For this review, take the finished solid that the model builds, in its own axes (mm). A direction names the side the tool comes from. Round coordinates to 2 decimals unless told otherwise and drop trailing zeros. Write each loop counter-clockwise with the first axis right and the second up, starting at its lowest first coordinate (ties: lowest second). Pieces come first, ordered by that corner, then holes. Notation, with made-up numbers: (21, 82) -> (55, 82) arc R19 cw to (55, 96) -> close; hole circle Ø5 at (-35.5, -8). An arc over 180 degrees is marked (long way). Answer as CSV lines item,"result". Start each with the question number.
Item 1: Take a section at B-B on y = 3.5. Give the boundary of the cut face in (x, z).
Item 2: Mouldability with a two-part tool opening along Y and no side actions: class faces 6 (the cylindrical face through (-2.38, -0.01, 7.13)), 7 (the flat face through (0, 0, 9.525)), 8 (the flat face through (3, -0.635, 8)), 9 (the cylindrical face through (-0.2, -1.51, 2.54)) as +Y half, -Y half, draft (parallel to the pull), parting line (faces both ways), or undercut.
Item 3: For pin 1 Ø0.9 at (x, z) = (3.5, 8.5) entering from -Y (3 decimals); pin 2 Ø1.5 at (x, y) = (3, -2) entering from +Z; pin 3 Ø0.9 at (x, z) = (3, 7.5) entering from +Y (3 decimals), all flat-tipped, find the tip position at first contact; note any pin that passes through.
Item 4: Machinability: for faces 1 (the flat face through (0, 0, 5.159)), 2 (the flat face through (3, 0.635, 8)), 3 (the flat face through (-3, 0.635, 8)), 4 (the flat face through (-3, -0.635, 8)), 5 (the cylindrical face through (2.38, 0.01, 7.13)), which of the approach directions +Z, -Z, +X, -X, +Y, -Y give a long, thin tool a straight path to every point of the face, cutting with its end or side? Answer none if there is none.
Item 5: Wall thickness on probe 1 along Y at (x, z) = (0, 3.55) (3 decimals); probe 2 along Z at (x, y) = (3, 2); probe 3 along Z at (x, y) = (0, 2.5): over which ranges is each line inside the solid? List them lowest first. Write a range as from..to.
```python
from build123d import *
from build123d import SkipClean  # not in build123d's __all__

# Parameters (mm, degrees)
F0_R      = 4.15
F1_DEPTH  = 1.5875
F3_R      = 4.15
F4_DEPTH  = 1.5875
F6_R      = 2.38125
F7_DEPTH  = 1.5875
F9_DEPTH  = 3.175
F10_R     = 3.175
F11_DEPTH = 3.175
F12_R     = 1.524
F13_DEPTH = 5.159375


# Not quite as in the source:
# - after a boolean that leaves OpenCascade's solid faulty, fix() repairs it


with BuildPart() as f1:
    # F0 (on Top) → F1 (new body)
    with BuildSketch(Plane.XY):
        Circle(F0_R)
    extrude(amount=F1_DEPTH)



with BuildPart() as f4:
    # F3 (on offset) → F4 (new body)
    with BuildSketch(Plane.XY.offset(6.35)):
        Circle(F3_R)
    extrude(amount=-F4_DEPTH)



with BuildPart() as f7:
    # F6 (on offset) → F7 (new body)
    with BuildSketch(Plane.XY.offset(7.9375)):
        Circle(F6_R)
    extrude(amount=F7_DEPTH)


with BuildPart() as f4_1:
    add(f4.part, clean=False)

    add(f7.part)  # F9 merges F7
    # F8 (on face) → F9 (join, through all)
    with BuildSketch(Plane.XY.offset(6.35)):
        with BuildLine():
            Line((2.2950221268, -0.635), (4.1011309416, -0.635))
            ThreePointArc((4.1011309416, -0.635), (4.1377646989, -0.3184388422), (4.15, 0))
            ThreePointArc((4.15, 0), (4.1377646989, 0.3184388422), (4.1011309416, 0.635))
            Line((4.1011309416, 0.635), (2.2950221268, 0.635))
            ThreePointArc((2.2950221268, 0.635), (2.38125, 0), (2.2950221268, -0.635))
        make_face()
        with BuildLine():
            ThreePointArc((-4.1011309416, 0.635), (-4.15, 0), (-4.1011309416, -0.635))
            Line((-4.1011309416, -0.635), (-2.2950221268, -0.635))
            ThreePointArc((-2.2950221268, -0.635), (-2.38125, 0), (-2.2950221268, 0.635))
            Line((-2.2950221268, 0.635), (-4.1011309416, 0.635))
        make_face()
    extrude(amount=F9_DEPTH)

    add(f4_1.part.fix(), mode=Mode.REPLACE)


with BuildPart() as f1_1:
    add(f1.part, clean=False)

    add(f4_1.part)  # F11 merges F4
    # F10 (on face) → F11 (join, through all)
    with BuildSketch(Plane.XY.offset(1.5875)):
        Circle(F10_R)
    extrude(amount=F11_DEPTH)

    # F12 (on face) → F13 (cut)
    with BuildSketch(Plane(origin=(0, 0, 0), x_dir=(1, 0, 0), z_dir=(0, 0, -1))):
        Circle(F12_R)
    with SkipClean():  # cleaning this boolean's faces spoils the solid; the shape is the same uncleaned
        extrude(amount=-F13_DEPTH, mode=Mode.SUBTRACT)


solid = f1_1.part
```
Output values:
1,outline,"(-2.23, 0) -> (2.23, 0) -> (2.23, 1.59) -> (-2.23, 1.59) -> close; (-2.23, 4.76) -> (2.23, 4.76) -> (2.23, 6.35) -> (-2.23, 6.35) -> close"
2,face 6,"undercut"
2,face 7,"draft"
2,face 8,"-Y half"
2,face 9,"undercut"
3,pin 1,"stops at y = -0.635"
3,pin 2,"stops at z = 6.35"
3,pin 3,"stops at y = 0.635"
4,face 1,"-Z"
4,face 2,"+Z, +X, +Y"
4,face 3,"+Z, -X, +Y"
4,face 4,"+Z, -X, -Y"
4,face 5,"none"
5,probe 1,"y = -3.175..-1.524, 1.524..3.175"
5,probe 2,"z = 0..1.59, 4.76..6.35"
5,probe 3,"z = 0..6.35"
